from build123d import *

# Parameters (mm, degrees)
SKETCH1_W           = 40
SKETCH1_H           = 20
BOSS_EXTRUDE1_DEPTH = 40
SKETCH2_W           = 54.5
SKETCH2_H           = 3.2
BOSS_EXTRUDE2_DEPTH = 20
FILLET1_R           = 3
SKETCH3_R           = 2.95
BOSS_EXTRUDE3_DEPTH = 4.3
SCALE1_SCALE        = 1.025


with BuildPart() as part:
    # Sketch1 → Boss-Extrude1 (new body)
    with BuildSketch(Plane(origin=(0, 0, 0), x_dir=(1, 0, 0), z_dir=(0, 1, 0))):
        Rectangle(SKETCH1_W, SKETCH1_H)
    extrude(amount=BOSS_EXTRUDE1_DEPTH)

    # Sketch2 → Boss-Extrude2 (add)
    with BuildSketch(Plane.XY.offset(10)):
        with Locations((0, 29.3)):
            Rectangle(SKETCH2_W, SKETCH2_H)
    extrude(amount=-BOSS_EXTRUDE2_DEPTH)

    # Fillet1
    fillet1_edges = [part.edges().sort_by_distance(p)[0] for p in [
        (20, 13.85, 10),
        (-20, 13.85, 10),
        (-20, 13.85, -10),
        (20, 13.85, -10),
        (27.25, 29.3, 10),
        (27.25, 29.3, -10),
        (-27.25, 29.3, -10),
        (-27.25, 29.3, 10),
        (20, 35.45, 10),
        (-20, 35.45, 10),
        (-20, 35.45, -10),
        (20, 35.45, -10),
    ]]
    fillet(fillet1_edges, radius=FILLET1_R)

    # Sketch3 → Boss-Extrude3 (add)
    with BuildSketch(Plane(origin=(0, 40, 0), x_dir=(1, 0, 0), z_dir=(0, 1, 0))):
        with Locations(Location((10.2, 0, 0), (0, 0, 90))):
            Circle(SKETCH3_R)
    extrude(amount=BOSS_EXTRUDE3_DEPTH)


with BuildPart() as part_1:
    # Scale1: scaled about (0.036629402, 20.343175324, 0)
    add(part.part.scale(SCALE1_SCALE).moved(Location((-0.000915735, -0.508579383, 0))))


solid = part_1.part
Can you work these out from the model? Positions are in its coordinate system, mm. A direction names the side the tool comes from. Coordinates: 2 decimals unless noted, no trailing zeros. Write each loop counter-clockwise with the first axis right and the second up, starting at its lowest first coordinate (ties: lowest second). Pieces come first, ordered by that corner, then holes. Notation, with made-up numbers: M 14,6.5 L 39,6.5 A23 ccw 39,35.5 Z; hole C 71,84.25 d5. An arc over 180 degrees is marked long. Use one line per item in the form item = value.
Q1. For P1, Ø3, axis at x = -21.5, z = -3.5, coming from the +Y side; P2, Ø4.5, axis at y = 36.5, z = -3.5, coming from the -X side; P3, Ø1.5, axis at y = 13.5, z = -1, coming from the +X side, each with a flat end and sliding along its axis, tell me the tip position at first contact or that it passes through.
Model answer:
P1 = 40.49
P2 = -20.5
P3 = 20.5
Q2. I need wall thicknesses on line 1 along X through (y, z) = (9, -0.75); line 2 along Y through (x, z) = (4, -1); line 3 along Y through (x, z) = (22.5, 2). Which ranges of each line are inside material? Lowest first, please. Write a range as from..to.
Model answer:
line_1 = -20.5..20.5
line_2 = -0.51..40.49
line_3 = 27.88..31.16
Q3. If we section it at B-B (y = 34.5): Write out the boundary of the cut face in (x, z) (3 decimals), then the cut area to 3 significant figures.
Model answer:
outline = M -20.501,-7.175 A3.075 ccw -17.426,-10.25 L 17.424,-10.25 A3.075 ccw 20.499,-7.175 L 20.499,7.175 A3.075 ccw 17.424,10.25 L -17.426,10.25 A3.075 ccw -20.501,7.175 Z
area = 832 mm^2
Q4. If we section it at C-C (x = -16.5): Write out the boundary of the cut face in (y, z).
Model answer:
outline = M -0.51,-10.25 L 40.49,-10.25 L 40.49,10.25 L -0.51,10.25 Z
Q5. If we section it at D-D (z = 0): Write out the boundary of the cut face in (x, y).
Model answer:
outline = M -27.93,27.88 L -20.5,27.88 L -20.5,-0.51 L 20.5,-0.51 L 20.5,27.88 L 27.93,27.88 L 27.93,31.16 L 20.5,31.16 L 20.5,40.49 L 13.48,40.49 L 13.48,44.9 L 7.43,44.9 L 7.43,40.49 L -20.5,40.49 L -20.5,31.16 L -27.93,31.16 Z
Q6. If we section it at A-A (z = 6.5): Write out the boundary of the cut face in (x, y).
Model answer:
outline = M -27.93,27.88 L -20.5,27.88 L -20.5,-0.51 L 20.5,-0.51 L 20.5,27.88 L 27.93,27.88 L 27.93,31.16 L 20.5,31.16 L 20.5,40.49 L -20.5,40.49 L -20.5,31.16 L -27.93,31.16 Z
Q7. For faces 1 (the cylindrical face through (19.574, 13.886, 9.373)), 2 (the cylindrical face through (-19.58, 35.89, -9.37)), 3 (the cylindrical face through (13.406, 42.664, 0.655)), 4 (the cylindrical face through (19.574, 13.886, -9.373)), 5 (the flat face through (-20.501, 36, 0)), which set-ups out of +Z, -Z, +X, -X, +Y, -Y let a thin tool reach every point of the face, with its end or its side?
Model answer:
face_1 = +Z, +X, -Y
face_2 = -Z, -X, +Y
face_3 = +Y
face_4 = -Z, +X, -Y
face_5 = +Z, -Z, -X, +Y
